For this review, take the finished solid that the model builds, in its own axes (mm). Round coordinates to 2 decimals unless told otherwise and drop trailing zeros. Loops run counter-clockwise (first coordinate to the right, second up) from the corner with the lowest first, then second, coordinate; pieces in that order, holes last. Notation, with made-up numbers: M 39.5,29.5 L 64.5,29.5 A24 ccw 64.5,59.5 Z; hole C 3,26.25 d5. An arc over 180 degrees is marked long. One line per question, with ' | ' between items. Start each with the question number.
1) For probe 1 along X at (y, z) = (2.35, 0); probe 2 along Y at (x, z) = (-6.25, -9.5); probe 3 along Z at (x, y) = (8.89, 3.9), list the stretches that pass through material, from the lowest coordinate up. Write a range as from..to.
2) Mouldability with a two-part tool opening along X and no side actions: class faces 1 (the face through (5.5, 5.08, -0.2)), 2 (the face through (-0.41, 1.25, 7.33)), 3 (the face through (-0.661, 8.211, 5.037)) as pulls with the +X half, pulls with the -X half, needs draft (parallel to the pull), parting line crosses it, or undercut.
3) We need section A-A (x = 0). Give the boundary of the cut face in (y, z), and give its area (3 significant figures).
4) For pin 1 Ø6 at (y, z) = (8.5, 4) entering from +X; pin 2 Ø2 at (x, z) = (-6.5, -8) entering from +Y; pin 3 Ø1.6 at (x, y) = (0, 2.54) entering from +Z, all flat-tipped, find the tip position at first contact; note any pin that passes through.
5) We need section B-B (z = 0). Give the boundary of the cut face in (x, y), and give its area (3 significant figures).
6) We need section C-C (y = 10). Give the boundary of the cut face in (x, z), and give its area (3 significant figures).
7) We need section D-D (x = 8.89). Give the boundary of the cut face in (y, z), and give its area (3 significant figures).
Autodesk Inventor part; units mm, degrees
ref_plane "Work Plane1" through (0, 2.54, 12.7) normal (0, 0, 1) x (1, 0, 0)
ref_plane "YZ Plane" through (0, 0, 0) normal (1, 0, 0) x (0, 1, 0)
ref_plane "XZ Plane" through (0, 0, 0) normal (0, 1, 0) x (-1, 0, 0)
sketch "Sketch1" plane through (0, 0, 0) normal (0, 0, 1) x (1, 0, 0)
  line L0 (2.5, 11.43) -> (5.08, 11.43)
  line L1 (5.08, 11.43) -> (5.08, 5.08)
  line L2 (5.08, 5.08) -> (12.7, 5.08)
  line L3 (12.7, 5.08) -> (12.7, 0)
  line L4 (12.7, 0) -> (2.5, 0)
  line L5 (2.5, 0) -> (2.5, 11.43)
  line L6 (0, -2.286) -> (0, 13.716)
  point P0 (0, 0)
  dimension "d0" = 2.5
  dimension "d1" = 12.7
  dimension "d2" = 5.08
  dimension "d3" = 5.08
  dimension "d4" = 6.35
revolve "Revolution1" add sketch "Sketch1" angle 360 about axis through (0, -10, 0) along (0, 1, 0)
sketch "Sketch2" plane through (0, 5.08, 0) normal (0, 1, 0) x (1, 0, 0)
  circle A0 centre (0, 0) radius 12.7
  line L0 (-8.89, 0) -> (8.89, 0) construction
  dimension "d6" = 17.78
hole "Hole1" at (-8.89, 5.08, 0) at (8.89, 5.08, 0) direction (0, -1, 0) diameter 2.7051 end through all
ref_plane "Work Plane1" through (0, 2.54, 12.7) normal (0, 0, 1) x (1, 0, 0)
sketch "Sketch3" plane through (0, 2.54, 12.7) normal (0, 0, 1) x (1, 0, 0)
  point P0 (0, -2.54)
  point P1 (0, 0)
  dimension "d17" = 2.54
  dimension "d18" = 0
hole "Hole2" at (0, 2.54, 12.7) direction (0, 0, -1) diameter 2.7051 end up to surface
properties part number "carousel_hub"
Answers below:
1) probe 1: -12.7..-10.24, -7.54..-2.5, 2.5..7.54, 10.24..12.7 | probe 2: 0..5.08 | probe 3: -9.07..-1.35, 1.35..9.07
2) face 1: needs draft | face 2: undercut | face 3: parting line crosses it
3) outline: M 0,-12.7 L 5.08,-12.7 L 5.08,-5.08 L 11.43,-5.08 L 11.43,-2.5 L 0,-2.5 Z; M 0,2.5 L 1.19,2.5 L 1.19,12.7 L 0,12.7 Z; M 3.89,2.5 L 11.43,2.5 L 11.43,5.08 L 5.08,5.08 L 5.08,12.7 L 3.89,12.7 Z | area: 109 mm^2
4) pin 1: x = 4.98 | pin 2: y = 5.08 | pin 3: z = -2.37
5) outline: M -12.7,0 L -10.24,0 L -10.24,5.08 L -12.7,5.08 Z; M -7.54,0 L -2.5,0 L -2.5,11.43 L -5.08,11.43 L -5.08,5.08 L -7.54,5.08 Z; M 2.5,0 L 7.54,0 L 7.54,5.08 L 5.08,5.08 L 5.08,11.43 L 2.5,11.43 Z; M 10.24,0 L 12.7,0 L 12.7,5.08 L 10.24,5.08 Z | area: 109 mm^2
6) outline: C 0,0 d10.16; hole C 0,0 d5 | area: 61.4 mm^2
7) outline: M 0,-9.07 L 5.08,-9.07 L 5.08,-1.35 L 0,-1.35 Z; M 0,1.35 L 5.08,1.35 L 5.08,9.07 L 0,9.07 Z | area: 78.4 mm^2
